from build123d import *

# Parameters (mm, degrees)
SKETCH1_W           = 10.25
SKETCH1_H           = 10.9
BOSS_EXTRUDE1_DEPTH = 1.5
SKETCH2_W           = 6.39
SKETCH2_H           = 8.4
CUT_EXTRUDE1_DEPTH  = 8.630080275
SKETCH3_W           = 10.25
SKETCH3_H           = 10.9
SKETCH3_R           = 3.35
BOSS_EXTRUDE2_DEPTH = 13
BOSS_EXTRUDE3_DEPTH = 1


with BuildPart() as part:
    # Sketch1 → Boss-Extrude1 (new body)
    with BuildSketch(Plane(origin=(0, 0, 0), x_dir=(1, 0, 0), z_dir=(0, 1, 0))):
        Rectangle(SKETCH1_W, SKETCH1_H)
    extrude(amount=BOSS_EXTRUDE1_DEPTH)

    # Sketch2 → Cut-Extrude1 (cut, through all)
    with BuildSketch(Plane(origin=(0, 1.5, 0), x_dir=(1, 0, 0), z_dir=(0, 1, 0))):
        with Locations((0, -0.45)):
            Rectangle(SKETCH2_W, SKETCH2_H)
    extrude(amount=-CUT_EXTRUDE1_DEPTH, mode=Mode.SUBTRACT)

    # Sketch3 → Boss-Extrude2 (add)
    with BuildSketch(Plane(origin=(0, 1.5, 0), x_dir=(1, 0, 0), z_dir=(0, 1, 0))):
        Rectangle(SKETCH3_W, SKETCH3_H)
        with Locations(Location((0, -0.45, 0), (0, 0, 162.502742528))):
            Circle(SKETCH3_R, mode=Mode.SUBTRACT)
    extrude(amount=BOSS_EXTRUDE2_DEPTH)

    # Sketch5 → Boss-Extrude3 (add)
    with BuildSketch(Plane(origin=(0, 14.5, 0), x_dir=(1, 0, 0), z_dir=(0, 1, 0))):
        with BuildLine():
            Line((-5.75, 7.95), (-5.75, 7.3))
            ThreePointArc((-5.75, 7.3), (-6.262563133, 6.062563133), (-7.5, 5.55))
            Line((-7.5, 5.55), (-8.4, 5.55))
            Line((-8.4, 5.55), (-8.4, -5.45))
            Line((-8.4, -5.45), (-5.125, -5.45))
            Line((-5.125, -5.45), (-5.125, 5.45))
            Line((-5.125, 5.45), (5.125, 5.45))
            Line((5.125, 5.45), (5.125, -5.45))
            Line((5.125, -5.45), (8.4, -5.45))
            Line((8.4, -5.45), (8.4, 5.55))
            Line((8.4, 5.55), (7.5, 5.55))
            ThreePointArc((7.5, 5.55), (6.262563133, 6.062563133), (5.75, 7.3))
            Line((5.75, 7.3), (5.75, 7.95))
            Line((5.75, 7.95), (-5.75, 7.95))
        make_face()
    extrude(amount=-BOSS_EXTRUDE3_DEPTH)


solid = part.part
Part model, mm, in its own coordinate system. A direction names the side the tool comes from. Round coordinates to 2 decimals unless told otherwise and drop trailing zeros. Write each loop counter-clockwise with the first axis right and the second up, starting at its lowest first coordinate (ties: lowest second). Pieces come first, ordered by that corner, then holes. Notation, with made-up numbers: M -21,39 L 7,39 A14 ccw 7,55 Z; hole C 35.5,5.5 d11. An arc over 180 degrees is marked long. Return JSON: item names as keys, results as strings. Group by question number.
(1) Saw through at C-C on z = 0.45. Write the cut outline in (x, y) (3 decimals).
(2) Pin check, flat tips, straight feed: pin 1 Ø2 at (x, y) = (-1.5, 3.5) entering from -Z; pin 2 Ø8 at (y, z) = (9, -4) entering from +X (3 decimals); pin 3 Ø5.5 at (x, z) = (0, 0.45) entering from +Y; pin 4 Ø2.5 at (x, z) = (-1.5, 3.5) entering from -Y. Stop position of each tip, or through.
(3) Saw through at D-D on x = 4. Write the cut outline in (y, z).
(4) Two-plate mould, pull along X, no slides. Class faces 6 (the face through (5.125, 7, 0)), 7 (the face through (-5.125, 7, 0)), 8 (the face through (-2, 14.5, -3)), 9 (the face through (-3.195, 1, 1)): +X half, -X half, draft (parallel to the pull), parting line (faces both ways), or undercut.
(5) Drill centre lines: probe 1 along Z at (x, y) = (0, 6.75); probe 2 along X at (y, z) = (7, 0.45) (3 decimals); probe 3 along Z at (x, y) = (-0.5, 0.5). Where is each one in solid material? Low to high.
(6) Saw through at B-B on y = 9.25. Write the cut outline in (x, z) (3 decimals).
(7) Saw through at A-A on x = 0. Write the cut outline in (y, z).
(8) Which spindle directions (+Z, -Z, +X, -X, +Y, -Y) get a long thin tool onto all of the face, cutting with end or side? Do faces 1 (the face through (3.195, 1, 1)), 2 (the face through (0, 14, -7.95)), 3 (the face through (8, 14, -5.55)), 4 (the face through (0, 7, -5.45)), 5 (the face through (-8, 14, -5.55)). Say none if no direction does.
Returned:
{
 "1": {"outline": "M -8.4,13.5 L -5.125,13.5 L -5.125,0 L -3.195,0 L -3.195,1.5 L -3.35,1.5 L -3.35,14.5 L -8.4,14.5 Z; M 3.195,0 L 5.125,0 L 5.125,13.5 L 8.4,13.5 L 8.4,14.5 L 3.35,14.5 L 3.35,1.5 L 3.195,1.5 Z"},
 "2": {"pin 1": "z = -5.45", "pin 2": "x = 5.125", "pin 3": "through", "pin 4": "y = 0"},
 "3": {"outline": "M 0,-5.45 L 13.5,-5.45 L 13.5,-7.95 L 14.5,-7.95 L 14.5,5.45 L 0,5.45 Z"},
 "4": {"face 6": "+X half", "face 7": "-X half", "face 8": "draft", "face 9": "undercut"},
 "5": {"probe 1": "-5.45 to -2.9, 3.8 to 5.45", "probe 2": "-5.125 to -3.35, 3.35 to 5.125", "probe 3": "-5.45 to -3.75, 4.65 to 5.45"},
 "6": {"outline": "M -5.125,-5.45 L 5.125,-5.45 L 5.125,5.45 L -5.125,5.45 Z; hole C 0,0.45 d6.7"},
 "7": {"outline": "M 0,-5.45 L 13.5,-5.45 L 13.5,-7.95 L 14.5,-7.95 L 14.5,-2.9 L 1.5,-2.9 L 1.5,-3.75 L 0,-3.75 Z; M 0,4.65 L 1.5,4.65 L 1.5,3.8 L 14.5,3.8 L 14.5,5.45 L 0,5.45 Z"},
 "8": {"face 1": "-Y", "face 2": "-Z, +X, -X, +Y, -Y", "face 3": "-Z, +X, +Y, -Y", "face 4": "-Z, +X, -X, -Y", "face 5": "-Z, -X, +Y, -Y"}
}
